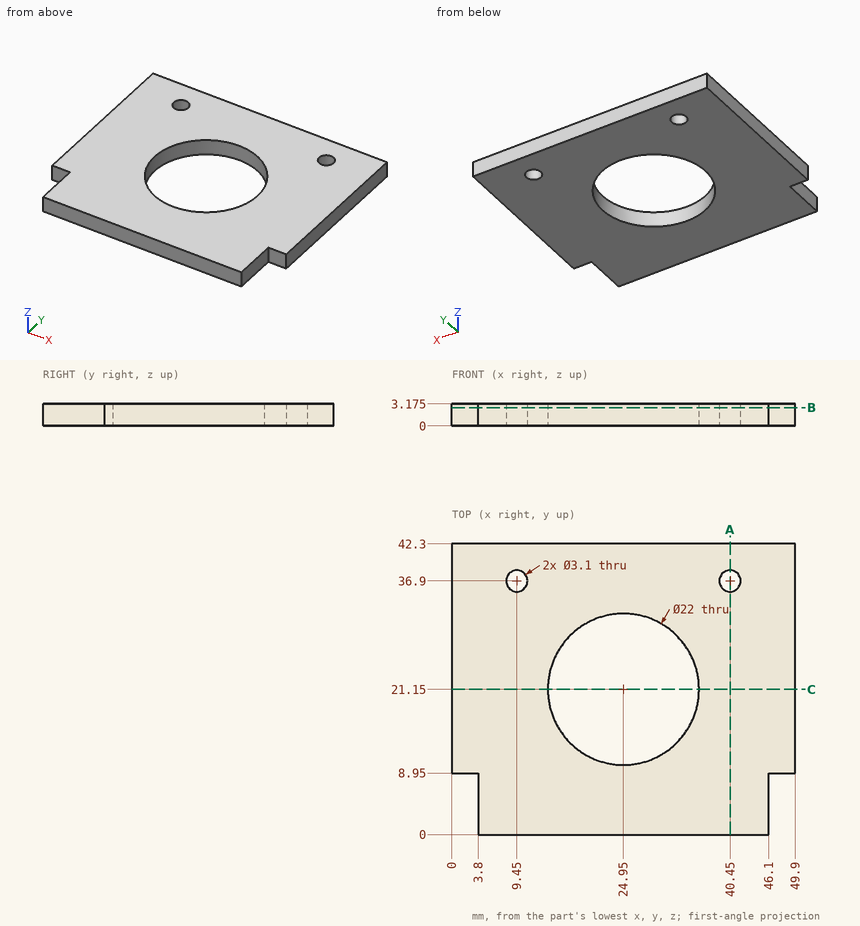
Print and shaded views of the part. All mm, measured from the part's lowest x, y and z. Coordinates: 2 decimals unless noted, no trailing zeros. Loops run counter-clockwise (first coordinate to the right, second up) from the corner with the lowest first, then second, coordinate; pieces in that order, holes last. Notation, with made-up numbers: (-2, 48.25) - (39, 48.25) arc R18 cw to (39, 60.25) - close; hole circle Ø8 at (42, 35). An arc over 180 degrees is marked (long way). Use one line per item in the form item = value. Start each with the question number.
1) Band-saw the part on B-B (z = 2.65). Give the cut face in (x, y).
2) Drill centre lines: L1, parallel to Y at x = 40.45, z = 1.15; L2, parallel to X at y = 3, z = 1.05; L3, parallel to X at y = 22, z = 1.05. Where is each one in solid material? Low to high. Write a range as from..to.
3) Band-saw the part on C-C (y = 21.15). Give the cut face in (x, z) (3 decimals).
4) Band-saw the part on A-A (x = 40.45). Give the cut face in (y, z) (3 decimals).
5) Flat gauge pins, fed straight in: pin 1 (1.6 mm diameter, centred on y = 5, z = 2, fed in from +X); pin 2 (1 mm diameter, centred on y = 6.5, z = 1, fed in from -X). Where does each tip first touch, or does it go through?
Check values:
q1.outline = (0, 8.95) - (3.8, 8.95) - (3.8, 0) - (46.1, 0) - (46.1, 8.95) - (49.9, 8.95) - (49.9, 42.3) - (0, 42.3) - close; hole circle Ø3.1 at (9.45, 36.9); hole circle Ø22 at (24.95, 21.15); hole circle Ø3.1 at (40.45, 36.9)
q2.L1 = 0..35.35, 38.45..42.3
q2.L2 = 3.8..46.1
q2.L3 = 0..13.98, 35.92..49.9
q3.outline = (0, 0) - (13.95, 0) - (13.95, 3.175) - (0, 3.175) - close; (35.95, 0) - (49.9, 0) - (49.9, 3.175) - (35.95, 3.175) - close
q4.outline = (0, 0) - (35.35, 0) - (35.35, 3.175) - (0, 3.175) - close; (38.45, 0) - (42.3, 0) - (42.3, 3.175) - (38.45, 3.175) - close
q5.pin_1 = 46.1
q5.pin_2 = 3.8
